Source: CAD feature listing. Evaluate the final solid. Frame: model axes, mm. Give positions to 0.01 mm unless a question says otherwise; leave off trailing zeros. Write each loop counter-clockwise with the first axis right and the second up, starting at its lowest first coordinate (ties: lowest second). Pieces come first, ordered by that corner, then holes. Notation, with made-up numbers: (-38, -19) -> (-25, -19) arc R23 ccw to (-25, -10) -> close; hole circle Ø5 at (-17.75, -37). An arc over 180 degrees is marked (long way). Write item = value, one per line.
from build123d import *

# Parameters (mm, degrees)
SKETCH1_R     = 1.7295
BASENUT_DEPTH = 1.7
CHAMFER1_SIZE = 0.17295


with BuildPart() as part:
    # Sketch1 → BaseNut (new body)
    with BuildSketch(Plane.XY):
        Polygon((2.020725942, -3.5), (4.041451884, 0), (2.020725942, 3.5), (-2.020725942, 3.5), (-4.041451884, 0), (-2.020725942, -3.5), align=None)
        Circle(SKETCH1_R, mode=Mode.SUBTRACT)
    extrude(amount=-BASENUT_DEPTH)

    # Sketch2 → Double-Chamfer (revolve, cut)
    with BuildSketch(Plane(origin=(0, 0, 0), x_dir=(1, 0, 0), z_dir=(0, 1, 0))):
        Polygon((-4.041451884, 1.7), (-3.5, 1.7), (-4.041451884, 1.554918405), align=None)
    revolve(axis=Axis((0, 0, -3.375940562), (0, 0, 1)), mode=Mode.SUBTRACT)

    # Chamfer1
    chamfer1_edges = [part.edges().sort_by_distance(p)[0] for p in [
        (-1.7295, 0, 0),
    ]]
    chamfer(chamfer1_edges, length=CHAMFER1_SIZE)


solid = part.part
1) Material intervals for L1, parallel to Y at x = 0, z = -0.95; L2, parallel to Y at x = -1.25, z = -0.45; L3, parallel to X at y = -0.5, z = -1.05, sorted ascending.
Computed:
L1 = -3.5 to -1.73, 1.73 to 3.5
L2 = -3.5 to -1.2, 1.2 to 3.5
L3 = -3.75 to -1.66, 1.66 to 3.75
2) Draft query along X for faces 1 (the flat face through (-3, 1.8, -0.8)), 2 (the conical face through (1.85, 3.19, -1.65)), 3 (the cylindrical face through (1.65, 0.52, -0.93)). Return one class per face: pulls with the +X half, pulls with the -X half, needs draft (parallel to the pull), parting line crosses it, or undercut.
Computed:
face_1 = pulls with the -X half
face_2 = pulls with the +X half
face_3 = undercut
3) Cut plane A-A (z = -0.3). Return the cut outline in (x, y).
Computed:
outline = (-4.04, 0) -> (-2.02, -3.5) -> (2.02, -3.5) -> (4.04, 0) -> (2.02, 3.5) -> (-2.02, 3.5) -> close; hole circle Ø3.46 at (0, 0)
4) Contact query for a flat-ended pin moving along its axis: pin 1 (3 mm diameter, centred on x = 0, y = 0, fed in from -Z). Output: stop coordinate, or through.
Computed:
pin_1 = through
